Verification items for the finished model (mm, model axes). A direction names the side the tool comes from. Coordinates: 2 decimals unless noted, no trailing zeros. Write each loop counter-clockwise with the first axis right and the second up, starting at its lowest first coordinate (ties: lowest second). Pieces come first, ordered by that corner, then holes. Notation, with made-up numbers: (50.25, 44.25) -> (69.25, 44.25) arc R12 cw to (69.25, 56.25) -> close; hole circle Ø1 at (86, 5). An arc over 180 degrees is marked (long way). Answer in a Markdown table with one row per item.
```python
from build123d import *

# Parameters (mm, degrees)
SKETCH_1_W             = 80
SKETCH_1_H             = 10
EXTRUDE_1_DEPTH        = 5
EXTRUDE_2_DEPTH        = 5
PATTERN_LINEAR_1_COUNT = 25
PATTERN_LINEAR_1_PITCH = 3.141592654
SKETCH_3_W             = 80
SKETCH_3_H             = 8
CUT_EXTRUDE_1_DEPTH    = 10
EXTRUDE_1_2_DEPTH      = 5
SKETCH_5_W             = 8
SKETCH_5_H             = 5
SKETCH_5_W_2           = 7.8
SKETCH_5_H_2           = 4.8
CUT_EXTRUDE_3_DEPTH    = 8
CHAMFER_1_SIZE         = 1


with BuildPart() as part:
    # 草图1 → Extrude 1 (new body)
    with BuildSketch(Plane.XY):
        with Locations((40, -5)):
            Rectangle(SKETCH_1_W, SKETCH_1_H)
    extrude(amount=EXTRUDE_1_DEPTH)

    # 草图2 → 拉伸2 (add)
    with BuildSketch(Plane.XY.offset(5)):
        Polygon((0, 0), (0.818933027, 2.25), (1.661788885, 2.25), (2.480721912, 0), align=None)
    extrude_2 = extrude(amount=-EXTRUDE_2_DEPTH)

    # 阵列(线性)1: 拉伸2 ×25
    with Locations(*[(i * PATTERN_LINEAR_1_PITCH, 0, 0) for i in range(1, PATTERN_LINEAR_1_COUNT)]):
        add(extrude_2)

    # 草图3 → 切除-拉伸1 (cut)
    with BuildSketch(Plane.XY.offset(5)):
        with Locations((40, -6)):
            Rectangle(SKETCH_3_W, SKETCH_3_H)
    extrude(amount=-CUT_EXTRUDE_1_DEPTH, mode=Mode.SUBTRACT)

    # 草图4 → Extrude 1 2 (add)
    with BuildSketch(Plane.XY.offset(5)):
        Polygon((80, 0), (84, 0), (84, 8), (92, 8), (92, 0), (92, -2), (80, -2), align=None)
    extrude(amount=-EXTRUDE_1_2_DEPTH)

    # 草图5 → 切除-拉伸3 (cut)
    with BuildSketch(Plane(origin=(0, 8, 0), x_dir=(1, 0, 0), z_dir=(0, 1, 0))):
        with Locations((88, -2.5)):
            Rectangle(SKETCH_5_W, SKETCH_5_H)
        with Locations((88, -2.5)):
            Rectangle(SKETCH_5_W_2, SKETCH_5_H_2, mode=Mode.SUBTRACT)
    extrude(amount=-CUT_EXTRUDE_3_DEPTH, mode=Mode.SUBTRACT)

    # 倒角1
    chamfer_1_edges = [part.edges().sort_by_distance(p)[0] for p in [
        (84.1, 8, 2.5),
        (91.9, 8, 2.5),
    ]]
    chamfer(chamfer_1_edges, length=CHAMFER_1_SIZE)


solid = part.part
```
1. Access from +Z, -Z, +X, -X, +Y, -Y to the whole of each face (thin tool, end or side, straight path). Record for faces 1 (the face through (68.04, 1.14, 2.54)), 2 (the face through (91.9, 4, 3)), 3 (the face through (88, 4, 0.1)).
Findings below:
| item | result |
|---|---|
| face 1 | +Z, -Z, +Y |
| face 2 | +Z, -Z, +X, +Y |
| face 3 | -Z, +X, +Y |
2. Release check for a two-part mould opening along X. For faces 4 (the face through (24.057, 1.141, 2.535)), 5 (the face through (88, 8, 3)), 6 (the face through (0, -1, 2)) record: released by +X, released by -X, zero draft, split by the parting line, or undercut.
Findings below:
| item | result |
|---|---|
| face 4 | undercut |
| face 5 | zero draft |
| face 6 | released by -X |
3. Sectioned sample at A-A, the plane y = 3.5. Record the cut outline in (x, z).
Findings below:
| item | result |
|---|---|
| outline | (84.1, 0.1) -> (91.9, 0.1) -> (91.9, 4.9) -> (84.1, 4.9) -> close |
4. Material ranges on probe 1 along Y at (x, z) = (69, 4.25); probe 2 along X at (y, z) = (6, 0.6); probe 3 along Y at (x, z) = (29.5, 1.35), recorded low to high. Write a range as from..to.
Findings below:
| item | result |
|---|---|
| probe 1 | y = -2..0 |
| probe 2 | x = 84.1..91.9 |
| probe 3 | y = -2..2.25 |
5. Go/stop test with flat-tipped pins: pin 1 (0.5 mm diameter, centred on x = 6, z = 3, fed in from +Y); pin 2 (1 mm diameter, centred on y = 6.5, z = 2, fed in from +X); pin 3 (0.7 mm diameter, centred on x = 51.5, z = 2, fed in from +Y). Record where each tip stops, or that it passes through.
Findings below:
| item | result |
|---|---|
| pin 1 | stops at y = 0 |
| pin 2 | stops at x = 91.9 |
| pin 3 | stops at y = 2.25 |
